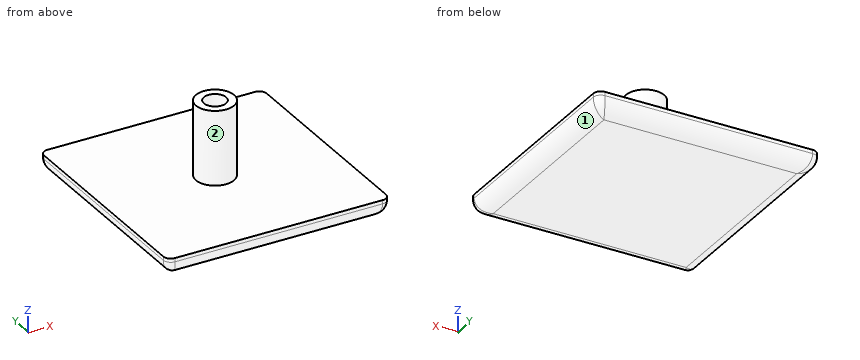
Autodesk Inventor part; units mm, degrees
ref_plane "YZ Plane" through (0, 0, 0) normal (1, 0, 0) x (0, 1, 0)
ref_plane "XZ Plane" through (0, 0, 0) normal (0, 1, 0) x (-1, 0, 0)
ref_plane "XY Plane" through (0, 0, 0) normal (0, 0, 1) x (1, 0, 0)
sketch "Náčrt1" plane through (0, 0, 0) normal (0, 0, 1) x (1, 0, 0)
  line L0 (0, 21) -> (0, -21)
  line L1 (-21, 0) -> (21, 0)
  line L2 (-15, 15) -> (15, 15)
  line L3 (15, 15) -> (15, -15)
  line L4 (15, -15) -> (-15, -15)
  line L5 (-15, -15) -> (-15, 15)
  point P0 (0, 0)
  dimension "d0" = 30
  dimension "d1" = 30
extrude "Vysunutí1" add sketch "Náčrt1" along normal blind 2.5
sketch "Náčrt2" plane through (0, 0, 2.5) normal (0, 0, 1) x (1, 0, 0)
  line L0 (-15, -15) -> (15, -15)
  line L1 (15, -15) -> (15, 15)
  line L2 (15, 15) -> (-15, 15)
  line L3 (-15, 15) -> (-15, -15)
  line L4 (0, 21) -> (0, -21)
  line L5 (-21, 0) -> (21, 0)
  circle A0 centre (0, 0) radius 2.575
  circle A1 centre (0, 0) radius 1.5
  dimension "d5" = 5.15
  dimension "d6" = 3
extrude "Vysunutí2" add sketch "Náčrt2" along normal blind 10 contours A0 L5 A1 L4 | L4 A1 L5 A0 | A0 L4 A1 L5 | L5 A1 L4 A0
fillet "Zaoblení1" radius 2 4 edges at (15, 0, 0) (0, 15, 0) (-15, 0, 0) (0, -15, 0)
fillet "Zaoblení2" radius 1 8 edges at (15, -15, 2.25) (14.4142, -14.4142, 0.5858) (15, 15, 2.25) (14.4142, 14.4142, 0.5858) (-15, 15, 2.25) (-14.4142, 14.4142, 0.5858) (-15, -15, 2.25) (-14.4142, -14.4142, 0.5858)
properties part number "záslepka"
The listing builds one solid part. Answer for the finished solid, in the listing's coordinates (mm). Face numbers are marked on the shaded views. A direction names the side the tool comes from. Give positions to 0.01 mm unless a question says otherwise; leave off trailing zeros. Write each loop counter-clockwise with the first axis right and the second up, starting at its lowest first coordinate (ties: lowest second). Pieces come first, ordered by that corner, then holes.
1) Find the intervals of material crossed by L1, parallel to Y at x = 0, z = 7.25 (3 decimals); L2, parallel to Z at x = 5, y = 13, in increasing order.
2) Section C-C (z = 7.25) is taken. Write down the section's boundary in (x, y) (3 decimals), and give its area (3 significant figures).
3) A tool of negligible diameter and unlimited length cuts with its end or side. For the marked faces 1 and 2, from which of +Z, -Z, +X, -X, +Y, -Y can it reach the whole face along a straight path? Write none if from no direction.
4) Section D-D (y = 5) is taken. Write down the section's boundary in (x, z).
5) Section A-A (y = 0) is taken. Write down the section's boundary in (x, z) (3 decimals), and give its area (3 significant figures).
6) Given P1, Ø1.8, axis at x = 0, y = 0, coming from the +Z side; P2, Ø1.5, axis at y = 4.5, z = 10.5, coming from the -X side, each flat-ended and moving along its own axis, determine where each tip first touches the part or whether it passes through.
Response:
1. L1: y = -2.575 to -1.5, 1.5 to 2.575
1. L2: z = 0 to 2.5
2. outline: circle Ø5.15 at (0, 0); hole circle Ø3 at (0, 0)
2. area: 13.8 mm2
3. face 1: -Z, +X, +Y, -Y
3. face 2: +Z
4. outline: (-15, 2) arc R2 ccw to (-13, 0) - (13, 0) arc R2 ccw to (15, 2) - (15, 2.5) - (-15, 2.5) - close
5. outline: (-15, 2) arc R2 ccw to (-13, 0) - (13, 0) arc R2 ccw to (15, 2) - (15, 2.5) - (2.575, 2.5) - (2.575, 12.5) - (1.5, 12.5) - (1.5, 2.5) - (-1.5, 2.5) - (-1.5, 12.5) - (-2.575, 12.5) - (-2.575, 2.5) - (-15, 2.5) - close
5. area: 94.8 mm2
6. P1: stops at z = 2.5
6. P2: passes through
